from build123d import *
from build123d.topology import SkipClean

# Parameters (mm, degrees)
ESQUISSE1_W        = 87
ESQUISSE1_H        = 140.4
BOSS_EXTRU_1_DEPTH = 150.6
ESQUISSE2_W        = 2.433761929
ESQUISSE2_H        = 5
ESQUISSE2_W_2      = 5
ESQUISSE2_H_2      = 2.433761929
ESQUISSE2_R        = 4
BOSS_EXTRU_5_DEPTH = 1.6
R_VOLUTION1_ANGLE  = 180
CHANFREIN1_SIZE    = 2.5
BOSS_EXTRU_6_DEPTH = 5


with BuildPart() as part:
    # Esquisse1 → Boss.-Extru.1 (new body)
    with BuildSketch(Plane(origin=(0, 0, 0), x_dir=(1, 0, 0), z_dir=(0, 1, 0))):
        Rectangle(ESQUISSE1_W, ESQUISSE1_H)
    extrude(amount=BOSS_EXTRU_1_DEPTH)

    # Esquisse2 → Boss.-Extru.5 (add)
    with BuildSketch(Plane.XY.offset(70.2)):
        with BuildLine():
            Line((-37.266238071, 100.9), (-37.266238071, 95.9))
            ThreePointArc((-37.266238071, 95.9), (-26.410438277, 71.989561723), (-2.5, 61.133761929))
            Line((-2.5, 61.133761929), (2.5, 61.133761929))
            ThreePointArc((2.5, 61.133761929), (26.410438277, 71.989561723), (37.266238071, 95.9))
            Line((37.266238071, 95.9), (37.266238071, 100.9))
            ThreePointArc((37.266238071, 100.9), (26.410438277, 124.810438277), (2.5, 135.666238071))
            Line((2.5, 135.666238071), (-2.5, 135.666238071))
            ThreePointArc((-2.5, 135.666238071), (-26.410438277, 124.810438277), (-37.266238071, 100.9))
        make_face()
        with Locations((38.483119036, 98.4)):
            Rectangle(ESQUISSE2_W, ESQUISSE2_H)
        with Locations((0, 136.883119036)):
            Rectangle(ESQUISSE2_W_2, ESQUISSE2_H_2)
        with Locations((-38.483119036, 98.4)):
            Rectangle(ESQUISSE2_W, ESQUISSE2_H)
        with Locations((0, 59.916880965)):
            Rectangle(ESQUISSE2_W_2, ESQUISSE2_H_2)
        with BuildLine():
            Line((-11, 45), (-28, 45))
            ThreePointArc((-28, 45), (-29.767766953, 44.267766953), (-30.5, 42.5))
            Line((-30.5, 42.5), (-30.5, 16.5))
            ThreePointArc((-30.5, 16.5), (-29.767766953, 14.732233047), (-28, 14))
            Line((-28, 14), (-11, 14))
            ThreePointArc((-11, 14), (-9.232233047, 14.732233047), (-8.5, 16.5))
            Line((-8.5, 16.5), (-8.5, 42.5))
            ThreePointArc((-8.5, 42.5), (-9.232233047, 44.267766953), (-11, 45))
        make_face()
        with Locations(Location((22.5, 29.5, 0), (0, 0, 180))):
            Circle(ESQUISSE2_R)
    extrude(amount=BOSS_EXTRU_5_DEPTH)

    # Esquisse3 → Révolution1 (revolve)
    with SkipClean():  # the faces are left unmerged after this step: merging them gives an invalid solid
        with BuildSketch(Plane.XY.offset(71.8)):
            with BuildLine():
                ThreePointArc((24.5, 29.5), (22.5, 31.5), (20.5, 29.5))
                Line((20.5, 29.5), (24.5, 29.5))
            make_face()
            with BuildLine():
                Line((24.5, 29.5), (20.5, 29.5))
                ThreePointArc((20.5, 29.5), (22.5, 27.5), (24.5, 29.5))
            make_face()
        revolve(axis=Axis((20.5, 29.5, 71.8), (1, 0, 0)), revolution_arc=R_VOLUTION1_ANGLE)

    # Chanfrein1
    # the kernel refuses this chamfer: 2.5 mm, written as the material it adds along each edge
    # the kernel refuses this chamfer: 2.5 mm, written as the material it takes off along each edge
    with BuildSketch(Plane(origin=(8.92920747, 58.7, 71.8), x_dir=(0, -0.027495876610587663, -0.9996219169112968), z_dir=(-1, 0, 0))) as chanfrein1_2_piece_1_section:
        Polygon((CHANFREIN1_SIZE * 0.999621916911, -CHANFREIN1_SIZE * 0.0274958766106), (-CHANFREIN1_SIZE * 0.0274958766106, -CHANFREIN1_SIZE * 0.999621916911), (0, 0), align=None)
    chanfrein1_2_piece_1 = extrude(amount=17.85841494, mode=Mode.PRIVATE)
    chanfrein1_2_piece_1 = split(chanfrein1_2_piece_1, bisect_by=Plane(origin=(2.719982047, 61.166365842, 70.2), z_dir=(0, 0, 1)), keep=Keep.TOP, mode=Mode.PRIVATE)
    add(chanfrein1_2_piece_1, mode=Mode.SUBTRACT)
    with BuildSketch(Plane(origin=(-39.7, 89.47079253, 71.8), x_dir=(-0.027495876610587663, 0, -0.9996219169112968), z_dir=(0, 1, 0))) as chanfrein1_2_piece_2_section:
        Polygon((CHANFREIN1_SIZE * 0.999621916911, -CHANFREIN1_SIZE * 0.0274958766106), (-CHANFREIN1_SIZE * 0.0274958766106, -CHANFREIN1_SIZE * 0.999621916911), (0, 0), align=None)
    chanfrein1_2_piece_2 = extrude(amount=17.85841494, mode=Mode.PRIVATE)
    chanfrein1_2_piece_2 = split(chanfrein1_2_piece_2, bisect_by=Plane(origin=(-37.233634158, 95.680017953, 70.2), z_dir=(0, 0, 1)), keep=Keep.TOP, mode=Mode.PRIVATE)
    add(chanfrein1_2_piece_2, mode=Mode.SUBTRACT)
    with BuildSketch(Plane(origin=(-8.92920747, 138.1, 71.8), x_dir=(0, 0.02749587661058214, -0.9996219169112969), z_dir=(1, 0, 0))) as chanfrein1_2_piece_3_section:
        Polygon((CHANFREIN1_SIZE * 0.999621916911, -CHANFREIN1_SIZE * 0.0274958766106), (-CHANFREIN1_SIZE * 0.0274958766106, -CHANFREIN1_SIZE * 0.999621916911), (0, 0), align=None)
    chanfrein1_2_piece_3 = extrude(amount=17.85841494, mode=Mode.PRIVATE)
    chanfrein1_2_piece_3 = split(chanfrein1_2_piece_3, bisect_by=Plane(origin=(-2.719982047, 135.633634158, 70.2), z_dir=(0, 0, 1)), keep=Keep.TOP, mode=Mode.PRIVATE)
    add(chanfrein1_2_piece_3, mode=Mode.SUBTRACT)
    with BuildSketch(Plane(origin=(39.7, 107.32920747, 71.8), x_dir=(0.027495876610587663, 0, -0.9996219169112968), z_dir=(0, -1, 0))) as chanfrein1_2_piece_4_section:
        Polygon((CHANFREIN1_SIZE * 0.999621916911, -CHANFREIN1_SIZE * 0.0274958766106), (-CHANFREIN1_SIZE * 0.0274958766106, -CHANFREIN1_SIZE * 0.999621916911), (0, 0), align=None)
    chanfrein1_2_piece_4 = extrude(amount=17.85841494, mode=Mode.PRIVATE)
    chanfrein1_2_piece_4 = split(chanfrein1_2_piece_4, bisect_by=Plane(origin=(37.233634158, 101.119982047, 70.2), z_dir=(0, 0, 1)), keep=Keep.TOP, mode=Mode.PRIVATE)
    add(chanfrein1_2_piece_4, mode=Mode.SUBTRACT)

    # Esquisse4 → Boss.-Extru.6 (add)
    with BuildSketch(Plane(origin=(0, 0, -70.2), x_dir=(-1, 0, 0), z_dir=(0, 0, -1))):
        with BuildLine():
            Line((-8, 15), (-8, 0))
            Line((-8, 0), (8, 0))
            Line((8, 0), (8, 15))
            ThreePointArc((8, 15), (5.656854249, 20.656854249), (0, 23))
            ThreePointArc((0, 23), (-5.656854249, 20.656854249), (-8, 15))
        make_face()
    extrude(amount=BOSS_EXTRU_6_DEPTH)


solid = part.part
Here's how the part is built. I have some questions about the finished solid (model axes, mm). A direction names the side the tool comes from. Coordinates: 2 decimals unless noted, no trailing zeros. Order: outer loops, then holes, each group sorted by start corner. A loop starts at its lowest first (then second) coordinate and runs counter-clockwise, first axis right, second up.
Item 1: If we section it at B-B on x = -14: List the corners of the cut face in (y, z) for me.
Result sheet:
outline: (0, -70.2) - (150.6, -70.2) - (150.6, 70.2) - (133.03, 70.2) - (133.03, 71.8) - (63.77, 71.8) - (63.77, 70.2) - (45, 70.2) - (45, 71.8) - (14, 71.8) - (14, 70.2) - (0, 70.2) - close
Item 2: For P1, Ø0.8, axis at y = 136.5, z = 71, coming from the -X side; P2, Ø1.5, axis at x = 28, y = 73, coming from the -Z side; P3, Ø5.5, axis at y = 10.5, z = -74, coming from the -X side, each with a flat end and sliding along its axis, tell me the tip position at first contact or that it passes through.
Result sheet:
P1: stops at x = -2.5
P2: stops at z = -70.2
P3: stops at x = -8
Item 3: If we section it at A-A on y = 12: List the corners of the cut face in (x, z) for me, plus the area to 3 significant figures.
Result sheet:
outline: (-43.5, -70.2) - (-8, -70.2) - (-8, -75.2) - (8, -75.2) - (8, -70.2) - (43.5, -70.2) - (43.5, 70.2) - (-43.5, 70.2) - close
area: 12,300 mm2
Item 4: If we section it at D-D on x = 5.5: List the corners of the cut face in (y, z) for me.
Result sheet:
outline: (0, -75.2) - (20.81, -75.2) - (20.81, -70.2) - (150.6, -70.2) - (150.6, 70.2) - (135.34, 70.2) - (135.34, 71.8) - (61.46, 71.8) - (61.46, 70.2) - (0, 70.2) - close
Item 5: For faces 1 (the face through (-1, 58, 70.2)), 2 (the face through (26.675, 124.543, 70.989)), 3 (the face through (8, 8, -73)), which set-ups out of +Z, -Z, +X, -X, +Y, -Y let a thin tool reach every point of the face, with its end or its side?
Result sheet:
face 1: +Z
face 2: +Z, +X, +Y
face 3: -Z, +X, +Y, -Y
Item 6: If we section it at C-C on y = 29.5: List the corners of the cut face in (x, z) for me.
Result sheet:
outline: (-43.5, -70.2) - (43.5, -70.2) - (43.5, 70.2) - (26.5, 70.2) - (26.5, 71.8) - (24.5, 71.8) arc R2 ccw to (20.5, 71.8) - (18.5, 71.8) - (18.5, 70.2) - (-8.5, 70.2) - (-8.5, 71.8) - (-30.5, 71.8) - (-30.5, 70.2) - (-43.5, 70.2) - close
Item 7: I need wall thicknesses on line 1 (Z direction, x = -18, y = 29.5); line 2 (Z direction, x = -34.5, y = 13.5). Which ranges of each line are inside material? Lowest first, please.
Result sheet:
line 1: z = -70.2 to 71.8
line 2: z = -70.2 to 70.2
